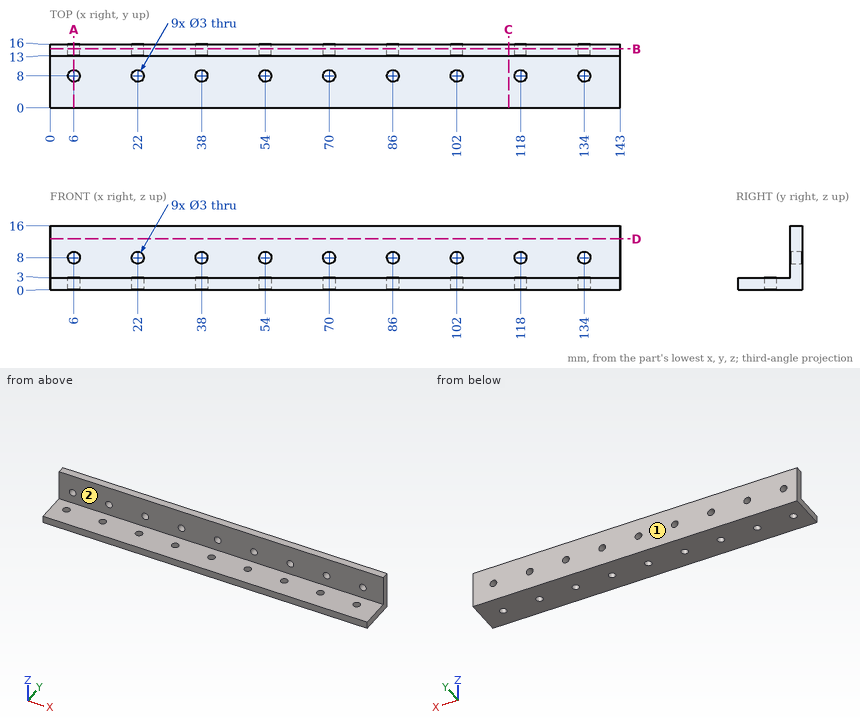
Geometry check sheet. Reference: drawing and pictorial views, mm from the part's lowest x, y, z. A direction names the side the tool comes from. Coordinates: 2 decimals unless noted, no trailing zeros. Loops run counter-clockwise (first coordinate to the right, second up) from the corner with the lowest first, then second, coordinate; pieces in that order, holes last. Notation, with made-up numbers: (-3, -37.5) - (40, -37.5) arc R16 cw to (40, -9.5) - close; hole circle Ø11 at (-20.75, -19.75). An arc over 180 degrees is marked (long way). Return JSON: item names as keys, results as strings.
1. Section check B-B, the plane y = 14.75. Count the separate pieces of the cut face and the enclosed holes in it, then the cut area to 3 significant figures.
Established:
{"separate pieces": "1", "enclosed holes": "9", "area": "2,220 mm2"}
2. Tool access check on the marked faces 1 and 2. Record the directions out of +Z, -Z, +X, -X, +Y, -Y that give a thin tool (end or side, any length) a straight path to the whole face; none if there is none.
Established:
{"face 1": "+Z, -Z, +X, -X, +Y", "face 2": "+Z, +X, -X, -Y"}
3. Thickness scan on L1, parallel to Y at x = 6, z = 1.4; L2, parallel to Z at x = 104, y = 9.25. Record the ranges inside material, lowest first.
Established:
{"L1": "y = 0 to 6.5, 9.5 to 16", "L2": "z = 0 to 3"}
4. Section check D-D, the plane z = 12.75. Record the boundary of the cut face in (x, y), then the cut area to 3 significant figures.
Established:
{"outline": "(0, 13) - (143, 13) - (143, 16) - (0, 16) - close", "area": "429 mm2"}
5. Go/stop test with flat-tipped pins: pin 1 (5 mm diameter, centred on x = 22, z = 8, fed in from -Y); pin 2 (5 mm diameter, centred on x = 121.5, y = 4, fed in from +Z). Record where each tip stops, or that it passes through.
Established:
{"pin 1": "stops at y = 13", "pin 2": "stops at z = 3"}
6. Section check C-C, the plane x = 115. Record the boundary of the cut face in (y, z), then the cut area to 3 significant figures.
Established:
{"outline": "(0, 0) - (16, 0) - (16, 16) - (13, 16) - (13, 3) - (0, 3) - close", "area": "87.0 mm2"}
7. Section check A-A, the plane x = 6. Record the boundary of the cut face in (y, z), then the cut area to 3 significant figures.
Established:
{"outline": "(0, 0) - (6.5, 0) - (6.5, 3) - (0, 3) - close; (9.5, 0) - (16, 0) - (16, 6.5) - (13, 6.5) - (13, 3) - (9.5, 3) - close; (13, 9.5) - (16, 9.5) - (16, 16) - (13, 16) - close", "area": "69.0 mm2"}
